Check sheet for the drawn part. Datum: minimum x, y, z corner. Units: mm. Give positions to 0.01 mm unless a question says otherwise; leave off trailing zeros. Write each loop counter-clockwise with the first axis right and the second up, starting at its lowest first coordinate (ties: lowest second). Pieces come first, ordered by that corner, then holes. Notation, with made-up numbers: M -29,78.5 L 29,78.5 A22 cw 29,94.5 Z; hole C 38,27.25 d8. An arc over 180 degrees is marked long. Write item = value, one per line. Start each with the question number.
1) Scan lines: L1, parallel to Z at x = 89, y = 2.6; L2, parallel to X at y = 2.5, z = 89; L3, parallel to X at y = 0.7, z = 23 (1 decimal). Record each from-to range of solid material in increasing order.
2) Sectioned sample at B-B, the plane z = 29.5. Record the cut outline in (x, y) (1 decimal), then the cut area to 3 significant figures.
3) Gauge pin test, flat ends, axial feed: pin 1 (1 mm diameter, centred on y = 1.5, z = 231, fed in from +X); pin 2 (1 mm diameter, centred on y = 1, z = 227, fed in from -X) (1 decimal); pin 3 (0.5 mm diameter, centred on x = 0.5, y = 2, fed in from +Z). Record the tip position at first contact, or that the pin passes through.
4) Sectioned sample at C-C, the plane x = 60. Record the cut outline in (y, z) (1 decimal).
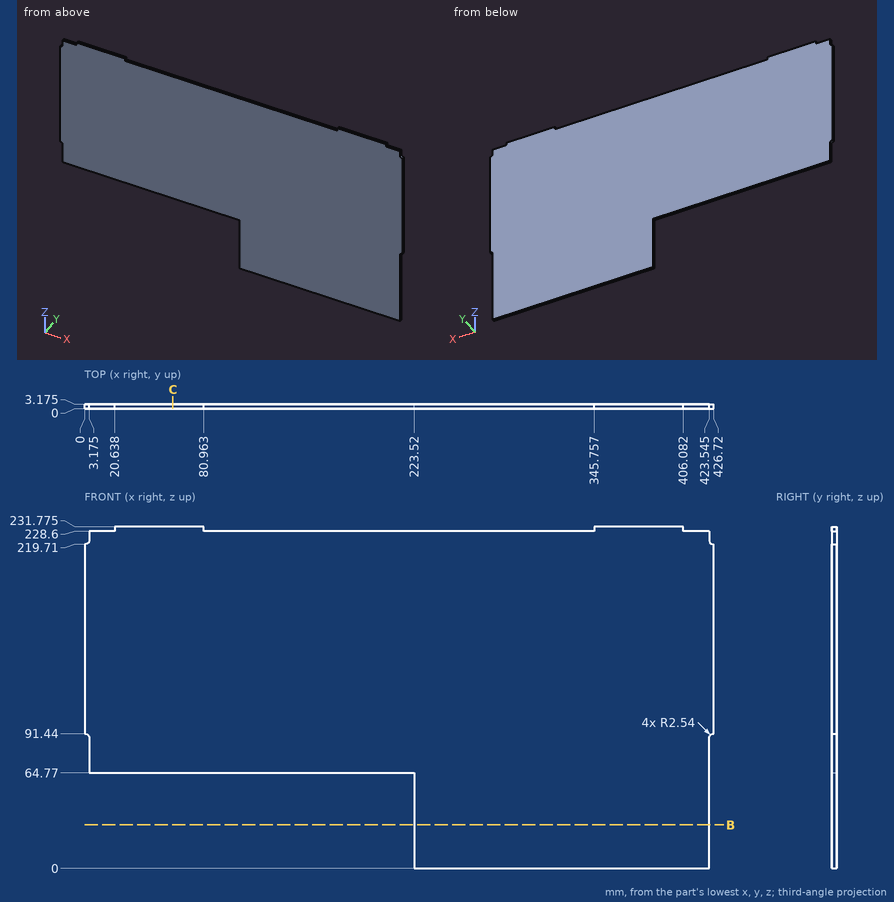
Data:
q1.L1 = 64.77 to 228.6
q1.L2 = 3.17 to 423.55
q1.L3 = 223.5 to 423.5
q2.outline = M 223.5,0 L 423.5,0 L 423.5,3.2 L 223.5,3.2 Z
q2.area = 635 mm2
q3.pin_1 = 406.08
q3.pin_2 = 3.2
q3.pin_3 = 219.71
q4.outline = M 0,64.8 L 3.2,64.8 L 3.2,231.8 L 0,231.8 Z
